Geometry check sheet. Reference: the model listing, model coordinates, mm. A direction names the side the tool comes from. Give positions to 0.01 mm unless a question says otherwise; leave off trailing zeros. Write each loop counter-clockwise with the first axis right and the second up, starting at its lowest first coordinate (ties: lowest second). Pieces come first, ordered by that corner, then holes. Notation, with made-up numbers: M 44.25,64 L 55.25,64 A23 cw 55.25,76 Z; hole C -17,25 d2. An arc over 180 degrees is marked long. One line per item, written item: value. Start each with the question number.
1. Release check for a two-part mould opening along X. For faces 1 (the face through (0, 12, -19)), 2 (the face through (25, 5, 0)), 3 (the face through (0, 17, 6)), 4 (the face through (8, 12, -29)) record: pulls with the +X half, pulls with the -X half, needs draft (parallel to the pull), parting line crosses it, or undercut.
2. Scan lines: line 1 (X direction, y = 16, z = -20.5); line 2 (Y direction, x = -23, z = 8.5); line 3 (Z direction, x = -7, y = 17.5). Record each from-to range of solid material in increasing order.
3. Cross-section at B-B on y = 21.25. Record the cut outline in (x, z).
4. Cross-section at D-D on x = 4.5. Record the cut outline in (y, z).
5. Tool access check on faces 5 (the face through (-22, 5, -16)), 6 (the face through (0, 5, 16)), 7 (the face through (21, 5, -16)), 8 (the face through (-8, 12, -29)). Record the directions out of +Z, -Z, +X, -X, +Y, -Y that give a thin tool (end or side, any length) a straight path to the whole face; none if there is none.
6. Gauge pin test, flat ends, axial feed: pin 1 (8 mm diameter, centred on x = -3, y = 11.5, fed in from -Z); pin 2 (5.5 mm diameter, centred on x = -22, y = 6, fed in from -Z); pin 3 (10 mm diameter, centred on y = 17, z = -28, fed in from +X). Record the tip position at first contact, or that the pin passes through.
7. Cross-section at A-A on z = -27.5. Record the cut outline in (x, y), then the cut area to 3 significant figures.
8. Cross-section at C-C on z = 0.5. Record the cut outline in (x, y), then the cut area to 3 significant figures.
from build123d import *

# Parameters (mm, degrees)
CROQUIS1_W                          = 50
CROQUIS1_H                          = 32
SALIENTE_EXTRUIR1_DEPTH             = 10
SALIENTE_EXTRUIR4_DEPTH             = 14
SALIENTE_EXTRUIR4_DIRECTION_2_REACH = 33.321


with BuildPart() as part:
    # Croquis1 → Saliente-Extruir1 (new body)
    with BuildSketch(Plane(origin=(0, 0, 0), x_dir=(1, 0, 0), z_dir=(0, 1, 0))):
        Rectangle(CROQUIS1_W, CROQUIS1_H)
    extrude(amount=SALIENTE_EXTRUIR1_DEPTH)

    # Croquis2 → Saliente-Extruir4 (add)
    with BuildSketch(Plane(origin=(0, 10, 0), x_dir=(1, 0, 0), z_dir=(0, 1, 0))):
        Polygon((-8, 39), (-18, 39), (-18, -6), (18, -6), (18, 39), (8, 39), (8, 19), (-8, 19), align=None)
    extrude(amount=SALIENTE_EXTRUIR4_DEPTH)

    # Saliente-Extruir4 direction 2: up to this face of the body (flat: up to its plane)
    saliente_extruir4_direction_2_end = Plane(part.part.faces().sort_by_distance((0, 0, 0))[0])
    # Croquis2 → Saliente-Extruir4 direction 2 (add, up to the picked face)
    with BuildSketch(Plane(origin=(0, 10, 0), x_dir=(1, 0, 0), z_dir=(0, 1, 0)), mode=Mode.PRIVATE) as saliente_extruir4_direction_2_sk1:
        Polygon((-8, 39), (-18, 39), (-18, -6), (18, -6), (18, 39), (8, 39), (8, 19), (-8, 19), align=None)
    saliente_extruir4_direction_2_tool1 = split(extrude(saliente_extruir4_direction_2_sk1.sketch, amount=-SALIENTE_EXTRUIR4_DIRECTION_2_REACH, mode=Mode.PRIVATE), bisect_by=saliente_extruir4_direction_2_end, keep=Keep.BOTH, mode=Mode.PRIVATE)
    add(saliente_extruir4_direction_2_tool1.solids().sort_by(Axis((0, 10, -13.423077), (0, -1, 0)))[0])


solid = part.part
Report:
1. face 1: undercut
1. face 2: pulls with the +X half
1. face 3: needs draft
1. face 4: undercut
2. line 1: x = -18 to -8, 8 to 18
2. line 2: y = 0 to 10
2. line 3: z = -19 to 6
3. outline: M -18,-39 L -8,-39 L -8,-19 L 8,-19 L 8,-39 L 18,-39 L 18,6 L -18,6 Z
4. outline: M 0,-19 L 24,-19 L 24,6 L 10,6 L 10,16 L 0,16 Z
5. face 5: -Z, -X, +Y, -Y
5. face 6: +Z, +X, -X, +Y, -Y
5. face 7: -Z, +X, +Y, -Y
5. face 8: -Z, +Y, -Y
6. pin 1: stops at z = -19
6. pin 2: stops at z = -16
6. pin 3: stops at x = 18
7. outline: M -18,0 L -8,0 L -8,24 L -18,24 Z; M 8,0 L 18,0 L 18,24 L 8,24 Z
7. area: 480 mm^2
8. outline: M -25,0 L 25,0 L 25,10 L 18,10 L 18,24 L -18,24 L -18,10 L -25,10 Z
8. area: 1,000 mm^2
